from build123d import *

# Parameters (mm, degrees)
BOSS_EXTRUDE1_DEPTH  = 5
M3_CLEARANCE_HOLE1_D = 3.4
CIRPATTERN1_COUNT    = 3


with BuildPart() as part:
    # Sketch2 → Boss-Extrude1 (new, symmetric)
    with BuildSketch(Plane.XY):
        Polygon((-87.988181024, 152.4), (-175.976362049, 0), (-87.988181024, -152.4), (87.988181024, -152.4), (175.976362049, 0), (87.988181024, 152.4), align=None)
    extrude(amount=BOSS_EXTRUDE1_DEPTH, both=True)

    # M3 Clearance Hole1 (through all)
    with Locations(Plane.XY.offset(5)):
        with Locations((-30.000000001, 115), (30.000000001, 115)):
            m3_clearance_hole1 = Hole(M3_CLEARANCE_HOLE1_D / 2)

    # CirPattern1: M3 Clearance Hole1 ×3 about axis
    cirpattern1_axis = Axis((0, 0, 0), (0, 0, 1))
    for i in range(1, CIRPATTERN1_COUNT):
        add(m3_clearance_hole1.rotate(cirpattern1_axis, i * 360 / CIRPATTERN1_COUNT), mode=Mode.SUBTRACT)


solid = part.part
Here's how the part is built. I have some questions about the finished solid (model axes, mm). Round coordinates to 2 decimals unless told otherwise and drop trailing zeros. Order: outer loops, then holes, each group sorted by start corner. A loop starts at its lowest first (then second) coordinate and runs counter-clockwise, first axis right, second up. Notation, with made-up numbers: (54.25, 45) -> (110.25, 45) arc R8 cw to (110.25, 52) -> close; hole circle Ø3 at (-26, -13). An arc over 180 degrees is marked (long way). Use CSV: the item, a comma, the result in double quotes.
1. I want a section at B-B on y = -15.5. List the corners of the cut face in (x, z) for me, and give its area (3 significant figures).
Recorded:
outline,"(-167.03, -5) -> (167.03, -5) -> (167.03, 5) -> (-167.03, 5) -> close"
area,"3,340 mm2"
2. I want a section at A-A on z = 0. List the corners of the cut face in (x, y) for me, and give its area (3 significant figures).
Recorded:
outline,"(-175.98, 0) -> (-87.99, -152.4) -> (87.99, -152.4) -> (175.98, 0) -> (87.99, 152.4) -> (-87.99, 152.4) -> close; hole circle Ø3.4 at (-114.59, -31.52); hole circle Ø3.4 at (-84.59, -83.48); hole circle Ø3.4 at (-30, 115); hole circle Ø3.4 at (30, 115); hole circle Ø3.4 at (84.59, -83.48); hole circle Ø3.4 at (114.59, -31.52)"
area,"80,400 mm2"
3. I'm going to push a flat-ended pin straight in: P1, Ø1, axis at x = -134.5, z = 1.5, coming from the +Y side. Where does the tip first touch, or does it pass through?
Recorded:
P1,"stops at y = 72.71"
4. I want a section at C-C on x = -139. List the corners of the cut face in (y, z) for me.
Recorded:
outline,"(-64.04, -5) -> (64.04, -5) -> (64.04, 5) -> (-64.04, 5) -> close"
5. I need wall thicknesses on line 1 along X through (y, z) = (115, 1); line 2 along Y through (x, z) = (-114, 2.25); line 3 along Y through (x, z) = (30, -1.5). Which ranges of each line are inside material? Lowest first, please.
Recorded:
line 1,"x = -109.58 to -31.7, -28.3 to 28.3, 31.7 to 109.58"
line 2,"y = -107.35 to -33.11, -29.93 to 107.35"
line 3,"y = -152.4 to 113.3, 116.7 to 152.4"
